from build123d import *

# Parameters (mm, degrees)
SKETCH1_R           = 1.5
SKETCH1_R_2         = 1.95
SKETCH1_R_3         = 3.9
BOSS_EXTRUDE1_DEPTH = 3.1


with BuildPart() as part:
    # Sketch1 → Boss-Extrude1 (new body)
    with BuildSketch(Plane.XY):
        with BuildLine():
            Line((0, 0), (0, 18.861213353))
            Line((0, 18.861213353), (18.442135624, 31.774535738))
            Line((18.442135624, 31.774535738), (26.642135624, 31.774535738))
            Line((26.642135624, 31.774535738), (47.552083318, 18.861213353))
            Line((47.552083318, 18.861213353), (47.552083318, 0))
            Line((47.552083318, 0), (30.440578527, -14.143422634))
            Line((30.440578527, -14.143422634), (30.440578527, -32.892135624))
            ThreePointArc((30.440578527, -32.892135624), (30.001238699, -33.952795796), (28.940578527, -34.392135624))
            Line((28.940578527, -34.392135624), (15.642135624, -34.392135624))
            ThreePointArc((15.642135624, -34.392135624), (14.581475452, -33.952795796), (14.142135624, -32.892135624))
            Line((14.142135624, -32.892135624), (14.142135624, -14.142135624))
            Line((14.142135624, -14.142135624), (0, 0))
        make_face()
        with Locations(Location((4.1, 16.058642392, 0), (0, 0, 180))):
            Circle(SKETCH1_R, mode=Mode.SUBTRACT)
        with Locations(Location((3.1, 4.378644873, 0), (0, 0, 180))):
            Circle(SKETCH1_R, mode=Mode.SUBTRACT)
        with Locations(Location((11.5, 9.430606677, 0), (0, 0, 180))):
            Circle(SKETCH1_R_2, mode=Mode.SUBTRACT)
        with Locations(Location((35.152083318, 9.430606677, 0), (0, 0, 180))):
            Circle(SKETCH1_R_3, mode=Mode.SUBTRACT)
        with Locations(Location((16.642135624, -31.892135624, 0), (0, 0, 180))):
            Circle(SKETCH1_R, mode=Mode.SUBTRACT)
        with Locations(Location((27.940578527, -31.892135624, 0), (0, 0, 180))):
            Circle(SKETCH1_R, mode=Mode.SUBTRACT)
        with Locations(Location((16.642135624, 9.430606677, 0), (0, 0, 180))):
            Circle(SKETCH1_R, mode=Mode.SUBTRACT)
        with Locations(Location((27.940578527, 9.430606677, 0), (0, 0, 180))):
            Circle(SKETCH1_R, mode=Mode.SUBTRACT)
        with Locations(Location((22.542135624, 28.274535738, 0), (0, 0, 180))):
            Circle(SKETCH1_R, mode=Mode.SUBTRACT)
        with Locations(Location((44.552083318, 2.5, 0), (0, 0, 180))):
            Circle(SKETCH1_R, mode=Mode.SUBTRACT)
        with Locations(Location((44.552083318, 16.361213353, 0), (0, 0, 180))):
            Circle(SKETCH1_R, mode=Mode.SUBTRACT)
        with BuildLine():
            Line((18.442135624, -14.432395526), (18.442135624, -27.642135624))
            ThreePointArc((18.442135624, -27.642135624), (18.588582233, -27.995689014), (18.942135624, -28.142135624))
            Line((18.942135624, -28.142135624), (25.640578527, -28.142135624))
            ThreePointArc((25.640578527, -28.142135624), (25.994131918, -27.995689014), (26.140578527, -27.642135624))
            Line((26.140578527, -27.642135624), (26.140578527, -14.345175543))
            ThreePointArc((26.140578527, -14.345175543), (26.175312874, -14.162069365), (26.274690017, -14.004403481))
            ThreePointArc((26.274690017, -14.004403481), (22.194770242, -4.756187266), (18.301117356, -14.084355132))
            ThreePointArc((18.301117356, -14.084355132), (18.405541961, -14.24463353), (18.442135624, -14.432395526))
        make_face(mode=Mode.SUBTRACT)
        with BuildLine():
            Line((16.792135624, 16.058642392), (27.790578527, 16.058642392))
            ThreePointArc((27.790578527, 16.058642392), (29.204792089, 16.64442883), (29.790578527, 18.058642392))
            Line((29.790578527, 18.058642392), (29.790578527, 21.258642392))
            ThreePointArc((29.790578527, 21.258642392), (29.204792089, 22.672855954), (27.790578527, 23.258642392))
            Line((27.790578527, 23.258642392), (16.792135624, 23.258642392))
            ThreePointArc((16.792135624, 23.258642392), (15.377922061, 22.672855954), (14.792135624, 21.258642392))
            Line((14.792135624, 21.258642392), (14.792135624, 18.058642392))
            ThreePointArc((14.792135624, 18.058642392), (15.377922061, 16.64442883), (16.792135624, 16.058642392))
        make_face(mode=Mode.SUBTRACT)
    extrude(amount=BOSS_EXTRUDE1_DEPTH)


solid = part.part
Check sheet for the modelled part. Datum: model origin and axes. Units: mm. A direction names the side the tool comes from. Round coordinates to 2 decimals unless told otherwise and drop trailing zeros. Order: outer loops, then holes, each group sorted by start corner. A loop starts at its lowest first (then second) coordinate and runs counter-clockwise, first axis right, second up.
Q1. Scan lines: L1, parallel to Y at x = 26, z = 0.8; L2, parallel to X at y = -18, z = 1; L3, parallel to Y at x = 20, z = 1.2. Record each from-to range of solid material in increasing order.
Filled sheet:
L1: y = -34.39 to -27.99, -6.23 to 16.06, 23.26 to 31.77
L2: x = 14.14 to 18.44, 26.14 to 30.44
L3: y = -34.39 to -28.14, -5.24 to 16.06, 23.26 to 31.77
Q2. Set-up check for faces 4 (the face through (15.394, 22.688, 1.528)), 5 (the face through (30.441, -23, 2)), 6 (the face through (24, 7, 0)): record each of +Z, -Z, +X, -X, +Y, -Y from which the full face is reachable in a straight line by a thin tool's end or side.
Filled sheet:
face 4: +Z, -Z
face 5: +Z, -Z, +X, -Y
face 6: -Z, +X, -X, +Y, -Y
Q3. Cross-section at A-A, the plane x = 12.5. Enter the section's corners in (y, z).
Filled sheet:
outline: (-12.5, 0) - (7.76, 0) - (7.76, 3.1) - (-12.5, 3.1) - close; (11.1, 0) - (27.61, 0) - (27.61, 3.1) - (11.1, 3.1) - close
Q4. Cross-section at B-B, the plane y = -12. Enter the section's corners in (x, z).
Filled sheet:
outline: (12, 0) - (17.03, 0) - (17.03, 3.1) - (12, 3.1) - close; (27.47, 0) - (33.03, 0) - (33.03, 3.1) - (27.47, 3.1) - close
Q5. Draft check along X on faces 1 (the face through (14.59, -33.96, 1.53)), 2 (the face through (29.19, 16.63, 1.53)), 3 (the face through (22, 31.775, 2)). Enter one of: pulls with the +X half, pulls with the -X half, needs draft (parallel to the pull), parting line crosses it, or undercut.
Filled sheet:
face 1: pulls with the -X half
face 2: undercut
face 3: needs draft
Q6. Cross-section at D-D, the plane x = 40.5. Enter the section's corners in (y, z).
Filled sheet:
outline: (-5.83, 0) - (23.22, 0) - (23.22, 3.1) - (-5.83, 3.1) - close
Q7. Depth check by flat-ended pin: P1, Ø1.6, axis at y = -27.5, z = 1.5, coming from the -X side; P2, Ø0.9, axis at y = -24, z = 1, coming from the +X side; P3, Ø1.5, axis at y = 22, z = 1.5, coming from the -X side; P4, Ø2.5, axis at x = 22.54, y = 28.27, coming from the +Z side (3 decimals). Enter the tip coordinate at first touch or a pass-through.
Filled sheet:
P1: stops at x = 14.14
P2: stops at x = 30.44
P3: stops at x = 3.41
P4: passes through
Q8. Cross-section at C-C, the plane z = 1. Give the number of separate pieces and of enclosed holes in the cut face, plus the area to 3 significant figures.
Filled sheet:
separate pieces: 1
enclosed holes: 13
area: 1,620 mm2
